Part model, mm, in its own coordinate system. Give positions to 0.01 mm unless a question says otherwise; leave off trailing zeros. Write each loop counter-clockwise with the first axis right and the second up, starting at its lowest first coordinate (ties: lowest second). Pieces come first, ordered by that corner, then holes. Notation, with made-up numbers: M -33.75,85 L 7.25,85 A15 ccw 7.25,101 Z; hole C 22,42 d3. An arc over 180 degrees is marked long. Write item = value, one per line. Start each with the question number.
from build123d import *

# Parameters (mm, degrees)
FILLET1_R       = 0.2
FILLET2_R       = 0.4
HEX_2_DEPTH     = 2
THDSCHPAT_COUNT = 29
THDSCHPAT_PITCH = 0.689655172


with BuildPart() as part:
    # BodySke → Base-Revolve (revolve)
    with BuildSketch(Plane.XY, mode=Mode.PRIVATE) as base_revolve_sk:
        Polygon((0, 0), (0, 3.5), (4, 3.5), (4, 2), (48.61, 2), (49, 1.61), (49, 0), align=None)
    revolve(base_revolve_sk.sketch.rotate(Axis((-31.75, 0, 0), (1, 0, 0)), 90), axis=Axis((-31.75, 0, 0), (1, 0, 0)))  # turned: the seam where the file's is

    # Fillet1
    fillet1_edges = [part.edges().sort_by_distance(p)[0] for p in [
        (4, 0, -2),
    ]]
    fillet(fillet1_edges, radius=FILLET1_R)

    # Fillet2
    fillet2_edges = [part.edges().sort_by_distance(p)[0] for p in [
        (0, 0, -3.5),
    ]]
    fillet(fillet2_edges, radius=FILLET2_R)

    # Sketch2 → Hex-PreBroach (revolve, cut)
    with BuildSketch(Plane.XY, mode=Mode.PRIVATE) as hex_prebroach_sk:
        Polygon((0, 1.51), (2, 1.51), (2.871798906, 0), (0, 0), align=None)
    revolve(hex_prebroach_sk.sketch.rotate(Axis((0, 0, 0), (1, 0, 0)), 90), axis=Axis((0, 0, 0), (1, 0, 0)), mode=Mode.SUBTRACT)  # turned: the seam where the file's is

    # Sketch3 → Hex 2 (cut)
    with BuildSketch(Plane(origin=(0, 0, 0), x_dir=(0, 0.5, 0.866025404), z_dir=(-1, 0, 0))):
        Polygon((0.871798906, 1.51), (-0.871798906, 1.51), (-1.743597813, 0), (-0.871798906, -1.51), (0.871798906, -1.51), (1.743597813, 0), align=None)
    extrude(amount=-HEX_2_DEPTH, mode=Mode.SUBTRACT)

    # ThdSchSke → ThreadSchematic (revolve, cut)
    with BuildSketch(Plane.XY, mode=Mode.PRIVATE) as threadschematic_sk:
        Polygon((29, -1.61), (28.72691906, -2), (28.72691906, -2.5), (29.27308094, -2.5), (29.27308094, -2), align=None)
    threadschematic = revolve(threadschematic_sk.sketch.rotate(Axis((-3.175, 0, 0), (1, 0, 0)), 270), axis=Axis((-3.175, 0, 0), (1, 0, 0)), mode=Mode.SUBTRACT)  # turned: the seam where the file's is

    # ThdSchPat: ThreadSchematic ×29
    with Locations(*[(i * THDSCHPAT_PITCH, 0, 0) for i in range(1, THDSCHPAT_COUNT)]):
        add(threadschematic, mode=Mode.SUBTRACT)


solid = part.part
Q1. Drop flat-ended pins along their axis: P1, Ø4, axis at x = 29.5, y = -2, coming from the -Z side; P2, Ø3, axis at x = 7, z = -1, coming from the -Y side; P3, Ø1, axis at y = 0.5, z = -2, coming from the +X side; P4, Ø3, axis at x = 38.5, z = 1.5, coming from the +Y side. Give the stop position or say it passes through.
Q2. Probe line 1 along X through (y, z) = (-2.25, -0.5); line 2 along Y through (x, z) = (35, 0.75); line 3 along X through (y, z) = (1.5, -0.25). List the from-to ranges inside material, lowest first.
Q3. Slice it at A-A (x = 11). Give the cut face in (y, z), and give its area (3 significant figures).
Working result:
q1.P1 = -2
q1.P2 = -2
q1.P3 = 49
q1.P4 = 2
q2.line_1 = 0 to 4
q2.line_2 = -1.75 to 1.75
q2.line_3 = 2 to 49
q3.outline = C 0,0 d4
q3.area = 12.6 mm2
